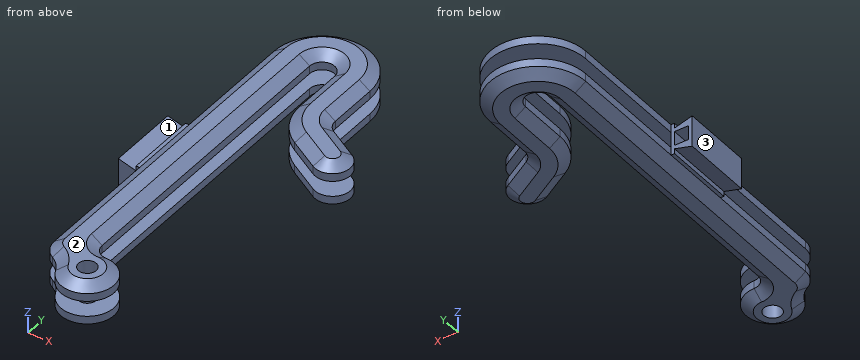
```python
from build123d import *
from OCP.BRepFilletAPI import BRepFilletAPI_MakeChamfer

# Parameters (mm, degrees)
SKETCH1_R           = 3.175
BOSS_EXTRUDE1_DEPTH = 16.51
FILLET1_R           = 10.16
CHAMFER1_SIZE       = 3.81
CHAMFER1_SIZE2      = 2.667790721
SPLIT1_START        = 5.503333164
SPLIT1_OUTLINE_R    = 3.175
SPLIT1_DEPTH        = 5.503333418
SKETCH4_W           = 11.174418558
SKETCH4_H           = 25.4
BOSS_EXTRUDE2_DEPTH = 12.7
SKETCH5_W           = 5.08
SKETCH5_H           = 11.174418558
CUT_EXTRUDE1_DEPTH  = 95.217988066
SKETCH7_W           = 5.08
SKETCH7_H           = 5.08
CUT_EXTRUDE2_DEPTH  = 20.32


# Read off the part's stored shape, not the designer's step: Split1
with BuildPart() as part:
    # Sketch1 → Boss-Extrude1 (new body)
    with BuildSketch(Plane.XY):
        with BuildLine():
            Line((4.445, 120.65), (4.445, 102.87))
            ThreePointArc((4.445, 102.87), (6.827068321, 93.98), (13.335, 87.472068321))
            Line((13.335, 87.472068321), (24.333522628, 81.122068321))
            ThreePointArc((24.333522628, 81.122068321), (33.007783942, 83.446329635), (30.683522628, 92.120590949))
            Line((30.683522628, 92.120590949), (19.685, 98.470590949))
            ThreePointArc((19.685, 98.470590949), (17.825590949, 100.33), (17.145, 102.87))
            Line((17.145, 102.87), (17.145, 120.65))
            ThreePointArc((17.145, 120.65), (0, 137.795), (-17.145, 120.65))
            Line((-17.145, 120.65), (-17.145, 7.62))
            ThreePointArc((-17.145, 7.62), (-14.913153673, 2.231846327), (-9.525, 0))
            ThreePointArc((-9.525, 0), (6.735192091, -6.735192091), (0, 9.525))
            ThreePointArc((0, 9.525), (-3.143089642, 10.826910358), (-4.445, 13.97))
            Line((-4.445, 13.97), (-4.445, 120.65))
            ThreePointArc((-4.445, 120.65), (0, 125.095), (4.445, 120.65))
        make_face()
        Circle(SKETCH1_R, mode=Mode.SUBTRACT)
    extrude(amount=BOSS_EXTRUDE1_DEPTH)

    # Fillet1
    fillet1_edges = [part.edges().sort_by_distance(p)[0] for p in [
        (-9.525, 0, 8.255),
    ]]
    fillet(fillet1_edges, radius=FILLET1_R)

    # Chamfer1: one chamfer whose edges measure the first distance from different faces: ONE call of the kernel's chamfer builder (chamfer() names one face for all edges)
    chamfer1_edges_1 = [part.edges().sort_by_distance(p)[0] for p in [
        (-3.143089642, 10.826910358, 16.51),
        (-4.445, 67.31, 16.51),
        (0, 125.095, 16.51),
        (4.445, 111.76, 16.51),
        (6.827068321, 93.98, 16.51),
        (18.834261314, 84.297068321, 16.51),
        (33.007783942, 83.446329635, 16.51),
        (25.184261314, 95.295590949, 16.51),
        (17.825590949, 100.33, 16.51),
        (7.990751239, -5.183967557, 16.51),
        (-10.525505779, -1.115347445, 16.51),
        (17.145, 111.76, 16.51),
        (-16.069536152, 3.716995189, 16.51),
        (0, 137.795, 16.51),
        (-17.145, 64.135, 16.51),
    ]]
    chamfer1_side_1 = [part.faces().sort_by_distance(p)[0] for p in [
        (-14.730576104, 4.515518933, 16.51),
    ]]
    chamfer1_edges_2 = [part.edges().sort_by_distance(p)[0] for p in [
        (-17.145, 64.135, 0),
        (0, 137.795, 0),
        (17.145, 111.76, 0),
        (17.825590949, 100.33, 0),
        (25.184261314, 95.295590949, 0),
        (33.007783942, 83.446329635, 0),
        (18.834261314, 84.297068321, 0),
        (6.827068321, 93.98, 0),
        (4.445, 111.76, 0),
        (0, 125.095, 0),
        (-4.445, 67.31, 0),
        (-3.143089642, 10.826910358, 0),
        (-16.069536152, 3.716995189, 0),
        (7.990751239, -5.183967557, 0),
        (-10.525505779, -1.115347445, 0),
    ]]
    chamfer1_side_2 = [part.faces().sort_by_distance(p)[0] for p in [
        (-14.730576104, 4.515518933, 0),
    ]]
    chamfer1 = BRepFilletAPI_MakeChamfer(part.part.solid().wrapped)
    for e in chamfer1_edges_1:
        chamfer1.Add(CHAMFER1_SIZE, CHAMFER1_SIZE2, e.wrapped, chamfer1_side_1[0].wrapped)  # the first distance lies on this face
    for e in chamfer1_edges_2:
        chamfer1.Add(CHAMFER1_SIZE, CHAMFER1_SIZE2, e.wrapped, chamfer1_side_2[0].wrapped)  # the first distance lies on this face
    add(Compound.cast(chamfer1.Shape()), mode=Mode.REPLACE)

    # Split1 outline → Split1 (cut)
    with BuildSketch(Plane.XY.offset(SPLIT1_START)):
        with BuildLine():
            ThreePointArc((-17.145, 7.62), (-16.069536152, 3.716995189), (-13.146720064, 0.915707063))
            ThreePointArc((-13.146720064, 0.915707063), (-10.525505779, -1.115347445), (-8.697909749, -3.882266219))
            ThreePointArc((-8.697909749, -3.882266219), (7.990751239, -5.183967557), (0, 9.525))
            ThreePointArc((0, 9.525), (-3.143089642, 10.826910358), (-4.445, 13.97))
            Line((-4.445, 13.97), (-4.445, 120.65))
            ThreePointArc((-4.445, 120.65), (0, 125.095), (4.445, 120.65))
            Line((4.445, 120.65), (4.445, 102.87))
            ThreePointArc((4.445, 102.87), (6.827068321, 93.98), (13.335, 87.472068321))
            Line((13.335, 87.472068321), (24.333522628, 81.122068321))
            ThreePointArc((24.333522628, 81.122068321), (33.007783942, 83.446329635), (30.683522628, 92.120590949))
            Line((30.683522628, 92.120590949), (19.685, 98.470590949))
            ThreePointArc((19.685, 98.470590949), (17.825590949, 100.33), (17.145, 102.87))
            Line((17.145, 102.87), (17.145, 120.65))
            ThreePointArc((17.145, 120.65), (0, 137.795), (-17.145, 120.65))
            Line((-17.145, 120.65), (-17.145, 7.62))
        make_face()
        Circle(SPLIT1_OUTLINE_R, mode=Mode.SUBTRACT)
    extrude(amount=SPLIT1_DEPTH, mode=Mode.SUBTRACT)

    # Sketch4 → Boss-Extrude2 (add)
    with BuildSketch(Plane.ZY.offset(17.145)):
        with Locations((8.255, 64.135)):
            Rectangle(SKETCH4_W, SKETCH4_H)
    extrude(amount=BOSS_EXTRUDE2_DEPTH)

    # Sketch5 → Cut-Extrude1 (cut, through all)
    with BuildSketch(Plane(origin=(0, 76.835, 0), x_dir=(1, 0, 0), z_dir=(0, 1, 0))):
        Polygon((-24.765, -2.667790721), (-18.414778652, -4.445000002), (-18.414778652, -2.667790721), align=None)
        with Locations((-27.305, -8.255)):
            Rectangle(SKETCH5_W, SKETCH5_H)
        Polygon((-18.415, -12.064999998), (-24.762176004, -13.842209279), (-18.415, -13.842209279), align=None)
    extrude(amount=-CUT_EXTRUDE1_DEPTH, mode=Mode.SUBTRACT)

    # Sketch7 → Cut-Extrude2 (cut)
    with BuildSketch(Plane(origin=(0, 76.835, 0), x_dir=(1, 0, 0), z_dir=(0, 1, 0))):
        with Locations((-20.955000002, -8.255)):
            Rectangle(SKETCH7_W, SKETCH7_H)
    extrude(amount=-CUT_EXTRUDE2_DEPTH, mode=Mode.SUBTRACT)


solid = part.part
```
Part model, mm, in its own coordinate system. Face numbers are marked on the shaded views. Round coordinates to 2 decimals unless told otherwise and drop trailing zeros. Write each loop counter-clockwise with the first axis right and the second up, starting at its lowest first coordinate (ties: lowest second). Pieces come first, ordered by that corner, then holes. Notation, with made-up numbers: (73, 30) -> (115, 30) arc R30 cw to (115, 56) -> close; hole circle Ø5 at (58.25, 29.25). An arc over 180 degrees is marked (long way). Return JSON: item names as keys, results as strings. Group by question number.
Q1. Pin check, flat tips, straight feed: pin 1 (1.5 mm diameter, centred on x = -20.5, y = 71.5, fed in from -Z); pin 2 (3 mm diameter, centred on y = 107.5, z = 4.5, fed in from +X) (3 decimals); pin 3 (2.5 mm diameter, centred on y = 65.5, z = 9.5, fed in from +X) (3 decimals). Stop position of each tip, or through.
Q2. Probe L1, parallel to Y at x = 0, z = 4.05 (3 decimals); L2, parallel to Y at x = 0, z = 15.25 (3 decimals); L3, parallel to X at y = 57, z = 10.5 (3 decimals). List the from-to ranges inside material, lowest first. Write a range as [from, to].
Q3. Mould opens along X. For the marked faces 1, 2 and 3 say: pulls with the +X half, pulls with the -X half, needs draft (parallel to the pull), parting line crosses it, or undercut.
Q4. Saw through at D-D on x = 23. Write the cut outline in (y, z).
Q5. Saw through at A-A on y = 47. Write the cut outline in (x, z) (3 decimals).
Q6. Saw through at C-C on z = 9. Write the cut outline in (x, y) (3 decimals), plus the area to 3 significant figures.
Answer:
{
 "1": {"pin 1": "z = 3.65", "pin 2": "x = 17.145", "pin 3": "x = -17.145"},
 "2": {"L1": "[-9.525, -3.175], [3.175, 9.525], [125.095, 137.795]", "L2": "[-7.514, -3.175], [3.175, 7.514], [127.106, 135.784]", "L3": "[-24.765, -23.495], [-18.415, -17.145]"},
 "3": {"face 1": "undercut", "face 2": "needs draft", "face 3": "pulls with the -X half"},
 "4": {"outline": "(81.89, 2.67) -> (86.29, 0) -> (92.16, 0) -> (96.56, 2.67) -> (96.56, 5.5) -> (81.89, 5.5) -> close; (81.89, 11.01) -> (96.56, 11.01) -> (96.56, 13.84) -> (92.16, 16.51) -> (86.29, 16.51) -> (81.89, 13.84) -> close"},
 "5": {"outline": "(-17.145, 2.668) -> (-13.335, 0) -> (-8.255, 0) -> (-4.445, 2.668) -> (-4.445, 5.503) -> (-17.145, 5.503) -> close; (-17.145, 11.007) -> (-4.445, 11.007) -> (-4.445, 13.842) -> (-8.255, 16.51) -> (-13.335, 16.51) -> (-17.145, 13.842) -> close"},
 "6": {"outline": "(-24.765, 51.435) -> (-17.145, 51.435) -> (-17.145, 76.835) -> (-18.415, 76.835) -> (-18.415, 56.515) -> (-23.495, 56.515) -> (-23.495, 76.835) -> (-24.765, 76.835) -> close", "area": "90.3 mm2"}
}
